Geometry check sheet. Reference: the model listing, model coordinates, mm. A direction names the side the tool comes from. Give positions to 0.01 mm unless a question says otherwise; leave off trailing zeros. Loops run counter-clockwise (first coordinate to the right, second up) from the corner with the lowest first, then second, coordinate; pieces in that order, holes last. Notation, with made-up numbers: (2, 63.5) -> (30, 63.5) arc R28 cw to (30, 93.5) -> close; hole circle Ø2 at (9.25, 7). An arc over 180 degrees is marked (long way). Write each question's results on one line, items separated by ' | '. Start each with the question number.
1) Set-up check for faces 4 (the face through (0, 8.585, -1)), 5 (the face through (-0.01, 7.47, 0.25)): record each of +Z, -Z, +X, -X, +Y, -Y from which the full face is reachable in a straight line by a thin tool's end or side.
2) Depth check by flat-ended pin: pin 1 (6 mm diameter, centred on y = -2.5, z = 4.5, fed in from -X). Enter the tip coordinate at first touch or a pass-through.
3) Sectioned sample at D-D on z = 0. Record the cut outline in (x, y).
4) Scan lines: line 1 (Z direction, x = 0, y = 6.75); line 2 (Y direction, x = -0.1, z = 0); line 3 (Y direction, x = 0.3, z = -4.5). Record each from-to range of solid material in increasing order. Write a range as from..to.
5) Sectioned sample at A-A on y = -5.5. Record the cut outline in (x, z), then the cut area to 3 significant figures.
6) Sectioned sample at C-C on x = 0. Record the cut outline in (y, z) (1 decimal).
7) Draft check along Y on faces 1 (the face through (0.01, 6.18, -3.34)), 2 (the face through (-0.006, 6.632, 1.42)), 3 (the face through (0, -7.5, 0.3)). Enter one of: pulls with the +Y half, pulls with the -Y half, needs draft (parallel to the pull), parting line crosses it, or undercut.
8) Sectioned sample at B-B on z = 5.25. Record the cut outline in (x, y).
```python
from build123d import *

# Parameters (mm, degrees)
BOSS_EXTRUDE1_DEPTH      = 0.4445
BOSS_EXTRUDE1_DEPTH_BACK = 0.4445
SKETCH3_R                = 0.5969
FILLET1_R                = 2.54
FILLET2_R                = 0.635
FILLET3_R                = 1.016


with BuildPart() as part:
    # Sketch3 → Boss-Extrude1 (new, two sides: drawn at the far end of the back side and taken through both)
    with BuildSketch(Plane(origin=(0, 0, 0), x_dir=(0, 0, -1), z_dir=(1, 0, 0)).offset(-BOSS_EXTRUDE1_DEPTH_BACK)):
        with BuildLine():
            Line((-2.2479, 8.584601843), (-3.258723069, 6.048738914))
            ThreePointArc((-3.258723069, 6.048738914), (0, -7.5057), (3.258723069, 6.048738914))
            Line((3.258723069, 6.048738914), (2.2479, 8.584601843))
            Line((2.2479, 8.584601843), (0.1905, 8.584601843))
            Line((0.1905, 8.584601843), (0.334067995, 5.845161304))
            ThreePointArc((0.334067995, 5.845161304), (0, -5.8547), (-0.334067995, 5.845161304))
            Line((-0.334067995, 5.845161304), (-0.1905, 8.584601843))
            Line((-0.1905, 8.584601843), (-2.2479, 8.584601843))
        make_face()
        with Locations((-1.290983998, 7.214881573)):
            Circle(SKETCH3_R, mode=Mode.SUBTRACT)
        with Locations((1.290983998, 7.214881573)):
            Circle(SKETCH3_R, mode=Mode.SUBTRACT)
    extrude(amount=BOSS_EXTRUDE1_DEPTH + BOSS_EXTRUDE1_DEPTH_BACK)

    # Fillet1
    fillet1_edges = [part.edges().sort_by_distance(p)[0] for p in [
        (0, 6.048738914, 3.258723069),
        (0, 6.048738914, -3.258723069),
    ]]
    fillet(fillet1_edges, radius=FILLET1_R)

    # Fillet2
    fillet2_edges = [part.edges().sort_by_distance(p)[0] for p in [
        (0, 5.845161304, 0.334067995),
        (0, 5.845161304, -0.334067995),
    ]]
    fillet(fillet2_edges, radius=FILLET2_R)

    # Fillet3
    fillet3_edges = [part.edges().sort_by_distance(p)[0] for p in [
        (0, 8.584601843, 2.2479),
        (0, 8.584601843, -2.2479),
    ]]
    fillet(fillet3_edges, radius=FILLET3_R)


solid = part.part
```
Result:
1) face 4: +Z, -Z, +X, -X, +Y | face 5: +X, -X
2) pin 1: x = -0.44
3) outline: (-0.44, -7.51) -> (0.44, -7.51) -> (0.44, -5.85) -> (-0.44, -5.85) -> close
4) line 1: -2.98..-1.67, -0.92..-0.29, 0.29..0.92, 1.67..2.98 | line 2: -7.51..-5.85 | line 3: -5.92..-3.75, 3.75..5.24
5) outline: (-0.44, -4.97) -> (0.44, -4.97) -> (0.44, -2.01) -> (-0.44, -2.01) -> close; (-0.44, 2.01) -> (0.44, 2.01) -> (0.44, 4.97) -> (-0.44, 4.97) -> close | area: 5.27 mm^2
6) outline: (5.7, -3.9) arc R2.5 cw to (6.9, -2.9) -> (7.9, -2.5) arc R1 ccw to (8.6, -1.6) -> (8.6, -0.2) -> (6.4, -0.3) arc R0.6 ccw to (5.8, -0.8) arc R5.9 cw (long way) to (5.8, 0.8) arc R0.6 ccw to (6.4, 0.3) -> (8.6, 0.2) -> (8.6, 1.6) arc R1 ccw to (7.9, 2.5) -> (6.9, 2.9) arc R2.5 cw to (5.7, 3.9) arc R7.2 ccw (long way) to start; hole circle Ø1.2 at (7.2, -1.3); hole circle Ø1.2 at (7.2, 1.3)
7) face 1: pulls with the +Y half | face 2: undercut | face 3: parting line crosses it
8) outline: (-0.44, -5.22) -> (0.44, -5.22) -> (0.44, -2.59) -> (-0.44, -2.59) -> close; (-0.44, 2.59) -> (0.44, 2.59) -> (0.44, 4.54) -> (-0.44, 4.54) -> close
